```python
from build123d import *

# Parameters (mm, degrees)
ESQUISSE1_R        = 2.5
ESQUISSE1_R_2      = 13.5
BOSS_EXTRU_1_DEPTH = 5


with BuildPart() as part:
    # Esquisse1 → Boss.-Extru.1 (new body)
    with BuildSketch(Plane(origin=(0, 0, 0), x_dir=(1, 0, 0), z_dir=(0, 1, 0))):
        Polygon((-12.5, 27.5), (-12.5, 22.5), (12.5, 22.5), (12.5, 27.5), (27.5, 27.5), (27.5, 12.5), (22.5, 12.5), (22.5, -7.5), (27.5, -7.5), (27.5, -27.5), (12.5, -27.5), (12.5, -22.5), (-12.5, -22.5), (-12.5, -27.5), (-27.5, -27.5), (-27.5, -7.5), (-22.5, -7.5), (-22.5, 12.5), (-27.5, 12.5), (-27.5, 27.5), align=None)
        with Locations(Location((17.5, 17.5, 0), (0, 0, 270))):
            Circle(ESQUISSE1_R, mode=Mode.SUBTRACT)
        with Locations(Location((-17.5, 17.5, 0), (0, 0, 90))):
            Circle(ESQUISSE1_R, mode=Mode.SUBTRACT)
        with Locations(Location((-17.5, -17.5, 0), (0, 0, 270))):
            Circle(ESQUISSE1_R, mode=Mode.SUBTRACT)
        with Locations(Location((17.5, -17.5, 0), (0, 0, 90))):
            Circle(ESQUISSE1_R, mode=Mode.SUBTRACT)
        with Locations(Location((0, 0, 0), (0, 0, 270))):
            Circle(ESQUISSE1_R_2, mode=Mode.SUBTRACT)
    extrude(amount=BOSS_EXTRU_1_DEPTH)


solid = part.part
```
Check sheet for the modelled part. Datum: model origin and axes. Units: mm. A direction names the side the tool comes from. Round coordinates to 2 decimals unless told otherwise and drop trailing zeros. Write each loop counter-clockwise with the first axis right and the second up, starting at its lowest first coordinate (ties: lowest second). Pieces come first, ordered by that corner, then holes. Notation, with made-up numbers: (26, -33.5) -> (42, -33.5) arc R24 ccw to (42, -8.5) -> close; hole circle Ø9 at (-8, 41.25). An arc over 180 degrees is marked (long way). One line per question, with ' | ' between items. Start each with the question number.
1. Sectioned sample at C-C, the plane z = 0. Record the cut outline in (x, y), then the cut area to 3 significant figures.
2. Sectioned sample at A-A, the plane x = -16. Record the cut outline in (y, z), then the cut area to 3 significant figures.
3. Set-up check for faces 4 (the face through (0, 2, -22.5)), 5 (the face through (17.4, 2.5, 20)), 6 (the face through (-22.5, 2, -2)), 7 (the face through (25, 2, 7.5)): record each of +Z, -Z, +X, -X, +Y, -Y from which the full face is reachable in a straight line by a thin tool's end or side.
4. Sectioned sample at B-B, the plane z = -17.5. Record the cut outline in (x, y), then the cut area to 3 significant figures.
5. Scan lines: line 1 along X through (y, z) = (3.2, -17.5); line 2 along X through (y, z) = (2.75, 0); line 3 along Z through (x, y) = (24, 2.8). Record each from-to range of solid material in increasing order. Write a range as from..to.
6. Depth check by flat-ended pin: pin 1 (4 mm diameter, centred on x = -17.5, z = -17.5, fed in from +Y); pin 2 (1.5 mm diameter, centred on y = 3.5, z = 1, fed in from -X); pin 3 (2 mm diameter, centred on x = -12.5, z = 3.5, fed in from +Y); pin 4 (1 mm diameter, centred on x = 9, y = 4, fed in from -Z). Enter the tip coordinate at first touch or a pass-through.
7. Sectioned sample at D-D, the plane x = 0. Record the cut outline in (y, z), then the cut area to 3 significant figures.
8. Release check for a two-part mould opening along X. For faces 1 (the face through (-12.5, 2, 25)), 2 (the face through (-25, 2, 7.5)), 3 (the face through (27.5, 2, -20)) record: +X half, -X half, draft (parallel to the pull), parting line (faces both ways), or undercut.
Taken from the geometry:
1) outline: (-22.5, 0) -> (-13.5, 0) -> (-13.5, 5) -> (-22.5, 5) -> close; (13.5, 0) -> (22.5, 0) -> (22.5, 5) -> (13.5, 5) -> close | area: 90.0 mm^2
2) outline: (0, -27.5) -> (5, -27.5) -> (5, -19.5) -> (0, -19.5) -> close; (0, -15.5) -> (5, -15.5) -> (5, 15.5) -> (0, 15.5) -> close; (0, 19.5) -> (5, 19.5) -> (5, 27.5) -> (0, 27.5) -> close | area: 235 mm^2
3) face 4: -Z, +Y, -Y | face 5: +Y, -Y | face 6: -X, +Y, -Y | face 7: +X, +Y, -Y
4) outline: (-27.5, 0) -> (-20, 0) -> (-20, 5) -> (-27.5, 5) -> close; (-15, 0) -> (15, 0) -> (15, 5) -> (-15, 5) -> close; (20, 0) -> (27.5, 0) -> (27.5, 5) -> (20, 5) -> close | area: 225 mm^2
5) line 1: x = -27.5..-20, -15..15, 20..27.5 | line 2: x = -22.5..-13.5, 13.5..22.5 | line 3: z = -27.5..-12.5, 7.5..27.5
6) pin 1: passes through | pin 2: stops at x = -22.5 | pin 3: stops at y = 5 | pin 4: stops at z = -22.5
7) outline: (0, -22.5) -> (5, -22.5) -> (5, -13.5) -> (0, -13.5) -> close; (0, 13.5) -> (5, 13.5) -> (5, 22.5) -> (0, 22.5) -> close | area: 90.0 mm^2
8) face 1: undercut | face 2: draft | face 3: +X half
